from build123d import *

# Parameters (mm, degrees)
SKETCH1_W                    = 412.496
SKETCH1_H                    = 152.4
BOSS_EXTRUDE1_DEPTH          = 4.7625
CUT_EXTRUDE2_START           = 4.7625
SKETCH2_R                    = 41.275
CUT_EXTRUDE2_DEPTH           = 225.688303193
F_5_16_18_TAPPED_HOLE1_D     = 6.5278
F_5_16_18_TAPPED_HOLE1_DEPTH = 9.525
F_5_16_18_TAPPED_HOLE1_TIP   = 1.961148974
F_5_16_18_TAPPED_HOLE2_D     = 6.5278
F_5_16_18_TAPPED_HOLE2_DEPTH = 9.525
F_5_16_18_TAPPED_HOLE2_TIP   = 1.961148974
F_5_16_18_TAPPED_HOLE3_D     = 6.5278
F_5_16_18_TAPPED_HOLE3_DEPTH = 9.525
F_5_16_18_TAPPED_HOLE3_TIP   = 1.961148974


with BuildPart() as part:
    # Sketch1 → Boss-Extrude1 (new, symmetric)
    with BuildSketch(Plane(origin=(0, 0, 0), x_dir=(1, 0, 0), z_dir=(0, 1, 0))):
        Rectangle(SKETCH1_W, SKETCH1_H)
    extrude(amount=BOSS_EXTRUDE1_DEPTH, both=True)

    # Sketch2 → Cut-Extrude2 (cut, through all)
    with BuildSketch(Plane(origin=(0, 0, 0), x_dir=(1, 0, 0), z_dir=(0, 1, 0)).offset(CUT_EXTRUDE2_START)):
        with Locations(Location((-130.048, 0, 0), (0, 0, 270))):
            Circle(SKETCH2_R)
        with Locations(Location((0, 0, 0), (0, 0, 270))):
            Circle(SKETCH2_R)
        with Locations(Location((130.048, 0, 0), (0, 0, 270))):
            Circle(SKETCH2_R)
    extrude(amount=-CUT_EXTRUDE2_DEPTH, mode=Mode.SUBTRACT)

    # 5/16-18 Tapped Hole1
    with Locations(Plane(origin=(0, 4.7625, 0), x_dir=(1, 0, 0), z_dir=(0, 1, 0))):
        with Locations((-166.0906, -36.0426), (-94.0054, -36.0426), (-166.0906, 36.0426), (-94.0054, 36.0426)):
            Hole(F_5_16_18_TAPPED_HOLE1_D / 2, depth=F_5_16_18_TAPPED_HOLE1_DEPTH)
            with Locations((0, 0, -(F_5_16_18_TAPPED_HOLE1_DEPTH + F_5_16_18_TAPPED_HOLE1_TIP / 2))):  # 118° drill point
                Cone(0, F_5_16_18_TAPPED_HOLE1_D / 2, F_5_16_18_TAPPED_HOLE1_TIP, mode=Mode.SUBTRACT)

    # 5/16-18 Tapped Hole2
    with Locations(Plane(origin=(0, 4.7625, 0), x_dir=(1, 0, 0), z_dir=(0, 1, 0))):
        with Locations((-36.0426, -36.0426), (36.0426, -36.0426), (-36.0426, 36.0426), (36.0426, 36.0426)):
            Hole(F_5_16_18_TAPPED_HOLE2_D / 2, depth=F_5_16_18_TAPPED_HOLE2_DEPTH)
            with Locations((0, 0, -(F_5_16_18_TAPPED_HOLE2_DEPTH + F_5_16_18_TAPPED_HOLE2_TIP / 2))):  # 118° drill point
                Cone(0, F_5_16_18_TAPPED_HOLE2_D / 2, F_5_16_18_TAPPED_HOLE2_TIP, mode=Mode.SUBTRACT)

    # 5/16-18 Tapped Hole3
    with Locations(Plane(origin=(0, 4.7625, 0), x_dir=(1, 0, 0), z_dir=(0, 1, 0))):
        with Locations((94.0054, -36.0426), (166.0906, -36.0426), (94.0054, 36.0426), (166.0906, 36.0426)):
            Hole(F_5_16_18_TAPPED_HOLE3_D / 2, depth=F_5_16_18_TAPPED_HOLE3_DEPTH)
            with Locations((0, 0, -(F_5_16_18_TAPPED_HOLE3_DEPTH + F_5_16_18_TAPPED_HOLE3_TIP / 2))):  # 118° drill point
                Cone(0, F_5_16_18_TAPPED_HOLE3_D / 2, F_5_16_18_TAPPED_HOLE3_TIP, mode=Mode.SUBTRACT)


solid = part.part
Verification items for the finished model (mm, model axes). Round coordinates to 2 decimals unless told otherwise and drop trailing zeros. Loops run counter-clockwise (first coordinate to the right, second up) from the corner with the lowest first, then second, coordinate; pieces in that order, holes last. Notation, with made-up numbers: (8.5, 23) - (55.5, 23) arc R28 cw to (55.5, 55) - close; hole circle Ø11 at (4, 10.25). An arc over 180 degrees is marked (long way). Use a Markdown table: item, result. Add a question column.
1. Section check B-B, the plane z = 0. Record the boundary of the cut face in (x, y) (1 decimal).
2. Gauge pin test, flat end, axial feed: pin 1 (10.5 mm diameter, centred on x = -94.01, z = -36.04, fed in from +Y). Record the tip position at first contact, or that the pin passes through.
3. Section check D-D, the plane x = 155.5. Record the boundary of the cut face in (y, z), plus the area to 3 significant figures.
4. Thickness scan on probe 1 along X at (y, z) = (-0.5, 0) (3 decimals); probe 2 along X at (y, z) = (-3, -15); probe 3 along Z at (x, y) = (129.5, 1). Record the ranges inside material, lowest first. Write a range as [from, to].
5. Section check A-A, the plane x = 0. Record the boundary of the cut face in (y, z) (1 decimal), plus the area to 3 significant figures.
6. Release check for a two-part mould opening along Z. For faces 1 (the face through (-3, 0, 76.2)), 2 (the face through (40.924, 0.067, -5.373)), 3 (the face through (89.755, 0.067, -8.948)), 4 (the face through (206.248, 0, 1)) record: released by +Z, released by -Z, zero draft, split by the parting line, or undercut.
7. Section check C-C, the plane y = 3. Give the number of separate pieces and of enclosed holes in the cut face, plus the area to 3 significant figures.
Checks:
| question | item | result |
|---|---|---|
| 1 | outline | (-206.2, -4.8) - (-171.3, -4.8) - (-171.3, 4.8) - (-206.2, 4.8) - close; (-88.8, -4.8) - (-41.3, -4.8) - (-41.3, 4.8) - (-88.8, 4.8) - close; (41.3, -4.8) - (88.8, -4.8) - (88.8, 4.8) - (41.3, 4.8) - close; (171.3, -4.8) - (206.2, -4.8) - (206.2, 4.8) - (171.3, 4.8) - close |
| 2 | pin 1 | stops at y = 4.76 |
| 3 | outline | (-4.76, -76.2) - (4.76, -76.2) - (4.76, -32.49) - (-4.76, -32.49) - close; (-4.76, 32.49) - (4.76, 32.49) - (4.76, 76.2) - (-4.76, 76.2) - close |
| 3 | area | 833 mm^2 |
| 4 | probe 1 | x = [-206.248, -171.323], [-88.773, -41.275], [41.275, 88.773], [171.323, 206.248] |
| 4 | probe 2 | x = [-206.25, -168.5], [-91.6, -38.45], [38.45, 91.6], [168.5, 206.25] |
| 4 | probe 3 | z = [-76.2, -41.27], [41.27, 76.2] |
| 5 | outline | (-4.8, -76.2) - (4.8, -76.2) - (4.8, -41.3) - (-4.8, -41.3) - close; (-4.8, 41.3) - (4.8, 41.3) - (4.8, 76.2) - (-4.8, 76.2) - close |
| 5 | area | 665 mm^2 |
| 6 | face 1 | released by +Z |
| 6 | face 2 | undercut |
| 6 | face 3 | undercut |
| 6 | face 4 | zero draft |
| 7 | separate pieces | 1 |
| 7 | enclosed holes | 15 |
| 7 | area | 46,400 mm^2 |
